Work out the finished part from the listing and answer in its coordinate system (mm). A direction names the side the tool comes from. Give positions to 0.01 mm unless a question says otherwise; leave off trailing zeros. Loops run counter-clockwise (first coordinate to the right, second up) from the corner with the lowest first, then second, coordinate; pieces in that order, holes last. Notation, with made-up numbers: M -32.75,71.25 L -0.75,71.25 A37 cw -0.75,108.25 Z; hole C 35,70 d2. An arc over 180 degrees is marked long. Use a Markdown table: item, result.
```python
from build123d import *

# Parameters (mm, degrees)
BOSS_EXTRUDE1_DEPTH = 4.7625
SKETCH5_R           = 3.5000057
CUT_EXTRUDE2_DEPTH  = 3.37125
CUT_EXTRUDE3_START  = 1.98
CUT_EXTRUDE3_DEPTH  = 1.98
SKETCH10_W          = 6.35
SKETCH10_H          = 0.79375
SKETCH10_W_2        = 35.745198541
SKETCH10_W_3        = 19.548012242
CUT_EXTRUDE4_DEPTH  = 68.70484365
CUT_EXTRUDE5_DEPTH  = 2.54
BOSS_EXTRUDE2_START = 2
BOSS_EXTRUDE2_DEPTH = 2
CUT_EXTRUDE6_DEPTH  = 62.875089873
BOSS_EXTRUDE4_REACH = 26.955
SKETCH15_W          = 13.3500114
SKETCH15_H          = 3.175
SKETCH15_W_2        = 4.031850112
SKETCH15_H_2        = 1.98
SKETCH20_W          = 13.3500114
SKETCH20_H          = 3.175
BOSS_EXTRUDE7_DEPTH = 3.175
SKETCH21_W          = 25.4
SKETCH21_H          = 31.75
BOSS_EXTRUDE8_DEPTH = 1.5875
FILLET1_R           = 3.175


with BuildPart() as part:
    # Sketch1 → Boss-Extrude1 (new body)
    with BuildSketch(Plane(origin=(0, 0, 0), x_dir=(1, 0, 0), z_dir=(0, 1, 0))):
        with BuildLine():
            Line((23.295952901, 15.613744639), (32.606191406, 26.334377035))
            ThreePointArc((32.606191406, 26.334377035), (32.033289602, 35.241600739), (23.119772343, 34.776777479))
            Line((23.119772343, 34.776777479), (-4.692006503, 4.278735207))
            ThreePointArc((-4.692006503, 4.278735207), (-6.274930424, -0.973523588), (-3.175, -5.499261314))
            Line((-3.175, -5.499261314), (27.78125, -23.371860585))
            ThreePointArc((27.78125, -23.371860585), (37.752424387, -26.756618196), (48.25987898, -26.067923237))
            ThreePointArc((48.25987898, -26.067923237), (49.382410995, -24.123640754), (47.438128512, -23.001108739))
            ThreePointArc((47.438128512, -23.001108739), (21.083895316, -12.623567162), (23.295952901, 15.613744639))
        make_face()
    extrude(amount=BOSS_EXTRUDE1_DEPTH)

    # Sketch5 → Cut-Extrude2 (cut)
    with BuildSketch(Plane.XZ):
        Circle(SKETCH5_R)
        with BuildLine():
            ThreePointArc((0, -3.5000057), (-3.5000057, 0), (0, 3.5000057))
            Line((0, 3.5000057), (-5.298345034, 3.5000057))
            ThreePointArc((-5.298345034, 3.5000057), (-6.35, 0), (-5.298345034, -3.5000057))
            Line((-5.298345034, -3.5000057), (0, -3.5000057))
        make_face()
    extrude(amount=-CUT_EXTRUDE2_DEPTH, mode=Mode.SUBTRACT)

    # Sketch6 → Cut-Extrude3 (cut)
    with BuildSketch(Plane.XZ.offset(-3.37125).offset(CUT_EXTRUDE3_START)):
        with BuildLine():
            Line((17.802786704, -2), (17.802786704, 2))
            Line((17.802786704, 2), (1.802786704, 3))
            ThreePointArc((1.802786704, 3), (3.5000057, 0), (1.802786704, -3))
            Line((1.802786704, -3), (17.802786704, -2))
        make_face()
    extrude(amount=-CUT_EXTRUDE3_DEPTH, mode=Mode.SUBTRACT)

    # Sketch10 → Cut-Extrude4 (cut, through all)
    with BuildSketch(Plane(origin=(-3.175, 0, 5.499261314), x_dir=(0.8660254037844385, 0, 0.5000000000000003), z_dir=(-0.5000000000000003, 0, 0.8660254037844385))):
        with Locations((-3.175, 4.365625)):
            Rectangle(SKETCH10_W, SKETCH10_H)
        with Locations((17.872599271, 4.365625)):
            Rectangle(SKETCH10_W_2, SKETCH10_H)
        with Locations((45.519204662, 4.365625)):
            Rectangle(SKETCH10_W_3, SKETCH10_H)
        with Locations((45.519204662, 0.396875)):
            Rectangle(SKETCH10_W_3, SKETCH10_H)
        with Locations((17.872599271, 0.396875)):
            Rectangle(SKETCH10_W_2, SKETCH10_H)
        with Locations((-3.175, 0.396875)):
            Rectangle(SKETCH10_W, SKETCH10_H)
    extrude(amount=-CUT_EXTRUDE4_DEPTH, mode=Mode.SUBTRACT)

    # Sketch11 → Cut-Extrude5 (cut)
    with BuildSketch(Plane.XZ.offset(-3.37125)):
        with BuildLine():
            Line((-5.298345034, 3.5000057), (0, 3.5000057))
            ThreePointArc((0, 3.5000057), (3.5000057, 0), (0, -3.5000057))
            Line((0, -3.5000057), (-5.298345034, -3.5000057))
            ThreePointArc((-5.298345034, -3.5000057), (-6.35, 0), (-5.298345034, 3.5000057))
        make_face()
    extrude(amount=-CUT_EXTRUDE5_DEPTH, mode=Mode.SUBTRACT)

    # Sketch12 → Boss-Extrude2 (add)
    with BuildSketch(Plane.XZ.offset(-0.79375).offset(BOSS_EXTRUDE2_START)):
        with BuildLine():
            Line((-3.175, 5.499261314), (-3.173710686, 5.5000057))
            Line((-3.173710686, 5.5000057), (0, 5.5000057))
            ThreePointArc((0, 5.5000057), (5.5000057, 0), (0, -5.5000057))
            Line((0, -5.5000057), (-3.57830535, -5.5000057))
            Line((-3.57830535, -5.5000057), (-4.692006503, -4.278735207))
            ThreePointArc((-4.692006503, -4.278735207), (-5.010327921, -3.901168303), (-5.298345034, -3.5000057))
            Line((-5.298345034, -3.5000057), (0, -3.5000057))
            ThreePointArc((0, -3.5000057), (3.5000057, 0), (0, 3.5000057))
            Line((0, 3.5000057), (-5.298345034, 3.5000057))
            ThreePointArc((-5.298345034, 3.5000057), (-4.353004683, 4.623186156), (-3.175, 5.499261314))
        make_face()
    extrude(amount=-BOSS_EXTRUDE2_DEPTH)

    # Sketch14 → Cut-Extrude6 (cut, through all)
    with BuildSketch(Plane(origin=(0, 3.96875, 0), x_dir=(1, 0, 0), z_dir=(0, 1, 0))):
        with BuildLine():
            Line((-2.50679919, 6.6750057), (18.4171905, 6.6750057))
            ThreePointArc((18.4171905, 6.6750057), (20.373146549, 11.408228546), (23.295952901, 15.613744639))
            Line((23.295952901, 15.613744639), (32.606191406, 26.334377035))
            ThreePointArc((32.606191406, 26.334377035), (32.033289602, 35.241600739), (23.119772343, 34.776777479))
            Line((23.119772343, 34.776777479), (-2.50679919, 6.6750057))
        make_face()
        with BuildLine():
            ThreePointArc((47.438128512, -23.001108739), (29.599662599, -20.753834653), (18.4171905, -6.6750057))
            Line((18.4171905, -6.6750057), (-1.138550987, -6.6750057))
            Line((-1.138550987, -6.6750057), (27.78125, -23.371860585))
            ThreePointArc((27.78125, -23.371860585), (37.752424387, -26.756618196), (48.25987898, -26.067923237))
            ThreePointArc((48.25987898, -26.067923237), (49.382410995, -24.123640754), (47.438128512, -23.001108739))
        make_face()
    extrude(amount=-CUT_EXTRUDE6_DEPTH, mode=Mode.SUBTRACT)

    # Sketch15 → Boss-Extrude4 (add, up to next)
    with BuildSketch(Plane(origin=(18.4171905, 0, 0), x_dir=(0, 0, -1), z_dir=(1, 0, 0)), mode=Mode.PRIVATE) as boss_extrude4_sk1:
        with Locations((0, 2.38125)):
            Rectangle(SKETCH15_W, SKETCH15_H)
        with Locations((0, 2.38125)):
            Rectangle(SKETCH15_W_2, SKETCH15_H_2, mode=Mode.SUBTRACT)
    boss_extrude4_tool1 = extrude(boss_extrude4_sk1.sketch, amount=-BOSS_EXTRUDE4_REACH, mode=Mode.PRIVATE) - part.part
    add(boss_extrude4_tool1.solids().sort_by_distance((18.41719, 2.38125, -6.537782))[0])

    # Sketch20 → Boss-Extrude7 (add)
    with BuildSketch(Plane(origin=(18.4171905, 0, 0), x_dir=(0, 0, -1), z_dir=(1, 0, 0))):
        with Locations((0, 2.38125)):
            Rectangle(SKETCH20_W, SKETCH20_H)
    extrude(amount=BOSS_EXTRUDE7_DEPTH)

    # Sketch21 → Boss-Extrude8 (add)
    with BuildSketch(Plane(origin=(0, 3.96875, 0), x_dir=(1, 0, 0), z_dir=(0, 1, 0))):
        with Locations((78.7421905, -19.05)):
            Rectangle(SKETCH21_W, SKETCH21_H)
        Polygon((91.4421905, 3.175), (21.5921905, 3.175), (21.5921905, -3.175), (66.0421905, -3.175), (91.4421905, -3.175), align=None)
    extrude(amount=-BOSS_EXTRUDE8_DEPTH)

    # Fillet1
    # the kernel refuses this fillet: 3.175 mm, written as the material it adds along each edge
    with BuildSketch(Plane(origin=(21.5921905, 3.96875, 3.175), x_dir=(0, 0, 1), z_dir=(0, -1, 0))) as fillet1_piece_1:
        with BuildLine():
            CenterArc((FILLET1_R, -FILLET1_R), FILLET1_R, 90, 90)
            Line((0, -FILLET1_R), (-FILLET1_R * 0.02, -FILLET1_R))
            Line((-FILLET1_R * 0.02, -FILLET1_R), (-FILLET1_R * 0.02, FILLET1_R * 0.02))
            Line((-FILLET1_R * 0.02, FILLET1_R * 0.02), (FILLET1_R, FILLET1_R * 0.02))
            Line((FILLET1_R, FILLET1_R * 0.02), (FILLET1_R, 0))
        make_face()
    extrude(amount=1.5875)
    with BuildSketch(Plane(origin=(21.5921905, 3.96875, -3.175), x_dir=(0, 0, -1), z_dir=(0, -1, 0))) as fillet1_piece_2:
        with BuildLine():
            CenterArc((FILLET1_R, FILLET1_R), FILLET1_R, 180, 90)
            Line((0, FILLET1_R), (-FILLET1_R * 0.02, FILLET1_R))
            Line((-FILLET1_R * 0.02, FILLET1_R), (-FILLET1_R * 0.02, -FILLET1_R * 0.02))
            Line((-FILLET1_R * 0.02, -FILLET1_R * 0.02), (FILLET1_R, -FILLET1_R * 0.02))
            Line((FILLET1_R, -FILLET1_R * 0.02), (FILLET1_R, 0))
        make_face()
    extrude(amount=1.5875)
    with BuildSketch(Plane(origin=(21.5921905, 2.38125, -3.175), x_dir=(0, -1, 0), z_dir=(0, 0, 1))) as fillet1_piece_3:
        with BuildLine():
            CenterArc((3.175, 2.749630657), FILLET1_R, 180, 60)
            Line((0, 2.749630657), (-0.0635, 2.749630657))
            Line((-0.0635, 2.749630657), (-0.0635, 0))
            Line((-0.0635, 0), (0, -0.0635))
            ThreePointArc((0, -0.0635), (0.79375, -0.0635), (1.55575, -0.054992613))
            Line((1.55575, -0.054992613), (1.5875, 0))
        make_face()
    extrude(amount=6.35)
    with BuildSketch(Plane(origin=(21.5921905, 3.96875, 3.175), x_dir=(0, 0, 1), z_dir=(0, -1, 0))) as fillet1_piece_4a_section:
        with BuildLine():
            CenterArc((FILLET1_R, -FILLET1_R), FILLET1_R, 90, 90)
            Line((0, -FILLET1_R), (-FILLET1_R * 0.02, -FILLET1_R))
            Line((-FILLET1_R * 0.02, -FILLET1_R), (-FILLET1_R * 0.02, FILLET1_R * 0.02))
            Line((-FILLET1_R * 0.02, FILLET1_R * 0.02), (FILLET1_R, FILLET1_R * 0.02))
            Line((FILLET1_R, FILLET1_R * 0.02), (FILLET1_R, 0))
        make_face()
    fillet1_piece_4a = extrude(amount=9.525, mode=Mode.PRIVATE)
    fillet1_piece_4a = split(fillet1_piece_4a, bisect_by=Plane(origin=(22.310994987, 0.79375, 3.893804488), z_dir=(0, 1, 0)), keep=Keep.TOP, mode=Mode.PRIVATE)
    fillet1_piece_4a = split(fillet1_piece_4a, bisect_by=Plane(origin=(22.310994987, 2.38125, 3.893804488), z_dir=(0, -1, 0)), keep=Keep.TOP, mode=Mode.PRIVATE)
    with BuildSketch(Plane(origin=(21.5921905, 2.38125, -3.175), x_dir=(0, -1, 0), z_dir=(0, 0, 1))) as fillet1_piece_4b_section:
        with BuildLine():
            CenterArc((3.175, 2.749630657), FILLET1_R, 180, 60)
            Line((0, 2.749630657), (-0.0635, 2.749630657))
            Line((-0.0635, 2.749630657), (-0.0635, 0))
            Line((-0.0635, 0), (0, -0.0635))
            ThreePointArc((0, -0.0635), (0.79375, -0.0635), (1.55575, -0.054992613))
            Line((1.55575, -0.054992613), (1.5875, 0))
        make_face()
    fillet1_piece_4b = extrude(amount=13.224076643, mode=Mode.PRIVATE)
    fillet1_piece_4b = split(fillet1_piece_4b, bisect_by=Plane(origin=(22.278976165, 1.970034442, 6.6750057), z_dir=(0, 0, -1)), keep=Keep.TOP, mode=Mode.PRIVATE)
    fillet1_piece_4b = split(fillet1_piece_4b, bisect_by=Plane(origin=(22.278976165, 1.970034442, 3.175), z_dir=(0, 0, 1)), keep=Keep.TOP, mode=Mode.PRIVATE)
    fillet1_piece_4 = fillet1_piece_4a & fillet1_piece_4b
    add(fillet1_piece_4)
    with BuildSketch(Plane(origin=(21.5921905, 2.38125, -10.049076643), x_dir=(0, -1, 0), z_dir=(0, 0, 1))) as fillet1_piece_5a_section:
        with BuildLine():
            CenterArc((3.175, 2.749630657), FILLET1_R, 180, 60)
            Line((0, 2.749630657), (-0.0635, 2.749630657))
            Line((-0.0635, 2.749630657), (-0.0635, 0))
            Line((-0.0635, 0), (0, -0.0635))
            ThreePointArc((0, -0.0635), (0.79375, -0.0635), (1.55575, -0.054992613))
            Line((1.55575, -0.054992613), (1.5875, 0))
        make_face()
    fillet1_piece_5a = extrude(amount=13.224076643, mode=Mode.PRIVATE)
    fillet1_piece_5a = split(fillet1_piece_5a, bisect_by=Plane(origin=(22.278976165, 1.970034442, -6.6750057), z_dir=(0, 0, 1)), keep=Keep.TOP, mode=Mode.PRIVATE)
    fillet1_piece_5a = split(fillet1_piece_5a, bisect_by=Plane(origin=(22.278976165, 1.970034442, -3.175), z_dir=(0, 0, -1)), keep=Keep.TOP, mode=Mode.PRIVATE)
    with BuildSketch(Plane(origin=(21.5921905, 3.96875, -3.175), x_dir=(0, 0, -1), z_dir=(0, -1, 0))) as fillet1_piece_5b_section:
        with BuildLine():
            CenterArc((FILLET1_R, FILLET1_R), FILLET1_R, 180, 90)
            Line((0, FILLET1_R), (-FILLET1_R * 0.02, FILLET1_R))
            Line((-FILLET1_R * 0.02, FILLET1_R), (-FILLET1_R * 0.02, -FILLET1_R * 0.02))
            Line((-FILLET1_R * 0.02, -FILLET1_R * 0.02), (FILLET1_R, -FILLET1_R * 0.02))
            Line((FILLET1_R, -FILLET1_R * 0.02), (FILLET1_R, 0))
        make_face()
    fillet1_piece_5b = extrude(amount=9.525, mode=Mode.PRIVATE)
    fillet1_piece_5b = split(fillet1_piece_5b, bisect_by=Plane(origin=(22.310994987, 0.79375, -3.893804488), z_dir=(0, 1, 0)), keep=Keep.TOP, mode=Mode.PRIVATE)
    fillet1_piece_5b = split(fillet1_piece_5b, bisect_by=Plane(origin=(22.310994987, 2.38125, -3.893804488), z_dir=(0, -1, 0)), keep=Keep.TOP, mode=Mode.PRIVATE)
    fillet1_piece_5 = fillet1_piece_5a & fillet1_piece_5b
    add(fillet1_piece_5)


solid = part.part
```
(1) A cutting plane is placed at A-A (z = 0). Write down the section's boundary in (x, y) (3 decimals), and give its area (3 significant figures).
Entries:
| item | result |
|---|---|
| outline | M 3.5,-1.206 L 5.5,-1.206 L 5.5,0.794 L 21.592,0.794 A3.175 cw 24.342,2.381 L 91.442,2.381 L 91.442,3.969 L 3.5,3.969 L 3.5,3.371 L 18.417,3.371 L 18.417,1.391 L 3.5,1.391 Z |
| area | 144 mm² |
(2) A cutting plane is placed at B-B (x = 43). Write down the section's boundary in (y, z) (3 decimals), and give its area (3 significant figures).
Entries:
| item | result |
|---|---|
| outline | M 2.381,-3.175 L 3.969,-3.175 L 3.969,3.175 L 2.381,3.175 Z |
| area | 10.1 mm² |
(3) Consider probe 1 along Z at (x, y) = (17.5, 3.25) (3 decimals); probe 2 along Z at (x, y) = (81, 2.7) (3 decimals); probe 3 along Y at (x, z) = (85, 17). Determine where each line is inside the solid, lowest interval first. Write a range as [from, to].
Entries:
| item | result |
|---|---|
| probe 1 | z = [-6.675, -2.019], [2.019, 6.675] |
| probe 2 | z = [-3.175, 34.925] |
| probe 3 | y = [2.38, 3.97] |
(4) Which of the six approach directions +Z, -Z, +X, -X, +Y, -Y give full straight-line access (tool end or side, diameter ignored) to faces 1 (the flat face through (-2, 0, 5.5)), 2 (the cylindrical face through (22.147, 2.756, 4.558)), 3 (the flat face through (73, 2.381, 11))?
Entries:
| item | result |
|---|---|
| face 1 | +Z, +X, -X, -Y |
| face 2 | +Z, +Y, -Y |
| face 3 | +Z, -Z, +X, -Y |
(5) Given P1, Ø0.6, axis at y = 2.5, z = 0.5, coming from the -X side; P2, Ø0.5, axis at y = 3, z = 19.5, coming from the -X side; P3, Ø1.8, axis at x = 7, z = 0, coming from the -Y side, each flat-ended and moving along its own axis, determine where each tip first touches the part or whether it passes through.
Entries:
| item | result |
|---|---|
| P1 | stops at x = 18.42 |
| P2 | stops at x = 66.04 |
| P3 | stops at y = 0.79 |
(6) The mould has two halves that part along Z. Classify faces 4 (the flat face through (10, 1.391, 0)), 5 (the cylindrical face through (5.5, -0.2, 0.1)), 6 (the flat face through (91.442, 3, 16)): released by +Z, released by -Z, zero draft, split by the parting line, or undercut.
Entries:
| item | result |
|---|---|
| face 4 | undercut |
| face 5 | split by the parting line |
| face 6 | zero draft |
(7) A cutting plane is placed at C-C (z = 32). Write down the section's boundary in (x, y), and give its area (3 significant figures).
Entries:
| item | result |
|---|---|
| outline | M 66.04,2.38 L 91.44,2.38 L 91.44,3.97 L 66.04,3.97 Z |
| area | 40.3 mm² |
